Can you work these out from the drawing? Everything is in mm from the part's minimum corner. A direction names the side the tool comes from. Coordinates: 2 decimals unless noted, no trailing zeros. Order: outer loops, then holes, each group sorted by start corner. A loop starts at its lowest first (then second) coordinate and runs counter-clockwise, first axis right, second up. Notation, with made-up numbers: (18, -20.5) - (43, -20.5) arc R17 ccw to (43, -11.5) - close; hole circle Ø1 at (-34, 23). An arc over 180 degrees is marked (long way). Answer as CSV lines item,"result". Start each with the question number.
Q1. I need wall thicknesses on line 1 (Y direction, x = 64, z = 0.55); line 2 (X direction, y = 6, z = 2); line 3 (X direction, y = 2.75, z = 3.05). Which ranges of each line are inside material? Lowest first, please.
Q2. For the marked faces 1, 2 and 3, which set-ups out of +Z, -Z, +X, -X, +Y, -Y let a thin tool reach every point of the face, with its end or its side?
Q3. For pin 1 Ø3.5 at (x, y) = (74.9, 7) entering from +Z; pin 2 Ø2.5 at (x, z) = (21, 1.5) entering from -Y; pin 3 Ø2 at (y, z) = (4.5, 1.5) entering from +X, each with a flat end and sliding along its axis, tell me the tip position at first contact or that it passes through.
Q4. Suppose I cut it at C-C (x = 60.5). Please give me the cut outline in (y, z), then the cut area to 3 significant figures.
Q5. Suppose I cut it at D-D (y = 2.75). Please give me the cut outline in (x, z).
Q6. Suppose I cut it at A-A (y = 7). Please give me the cut outline in (x, z).
Q7. Suppose I cut it at B-B (z = 4.05). Please give me the cut outline in (x, y), then the cut area to 3 significant figures.
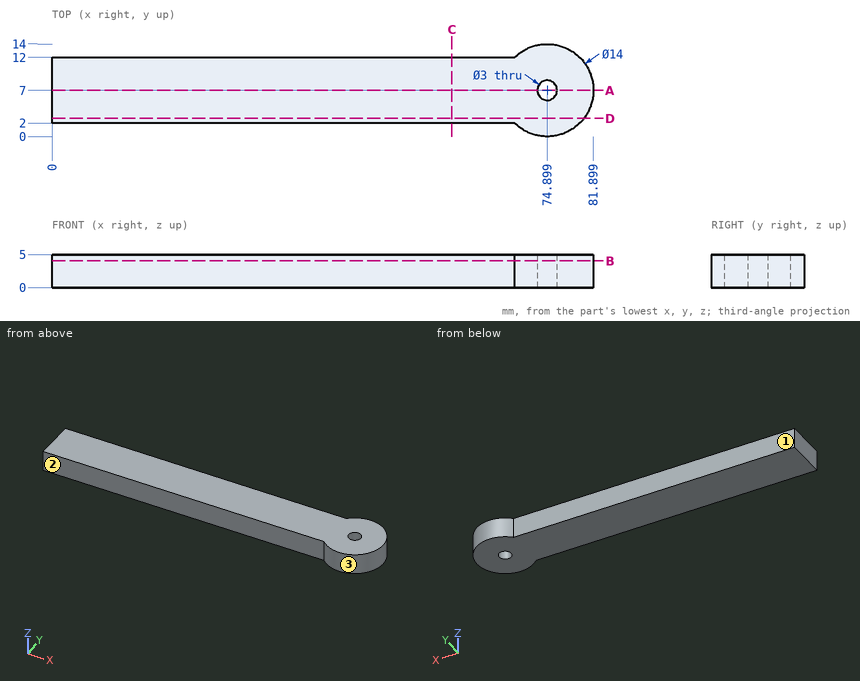
Here are the results:
1,line 1,"y = 2 to 12"
1,line 2,"x = 0 to 73.78, 76.02 to 81.83"
1,line 3,"x = 0 to 80.46"
2,face 1,"+Z, -Z, -X, +Y"
2,face 2,"+Z, -Z, -X, -Y"
2,face 3,"+Z, -Z"
3,pin 1,"stops at z = 5"
3,pin 2,"stops at y = 2"
3,pin 3,"stops at x = 81.74"
4,outline,"(2, 0) - (12, 0) - (12, 5) - (2, 5) - close"
4,area,"50.0 mm²"
5,outline,"(0, 0) - (80.46, 0) - (80.46, 5) - (0, 5) - close"
6,outline,"(0, 0) - (73.4, 0) - (73.4, 5) - (0, 5) - close; (76.4, 0) - (81.9, 0) - (81.9, 5) - (76.4, 5) - close"
7,outline,"(0, 2) - (70, 2) arc R7 ccw (long way) to (70, 12) - (0, 12) - close; hole circle Ø3 at (74.9, 7)"
7,area,"832 mm²"
